```python
from build123d import *

# Parameters (mm, degrees)
BOSS_EXTRUDE1_DEPTH   = 4.7625
F_6_CLEARANCE_HOLE1_D = 4.3053


with BuildPart() as part:
    # Sketch1 → Boss-Extrude1 (new body)
    with BuildSketch(Plane.XY):
        with BuildLine():
            Line((-3103.698757178, 1002.345694712), (-3103.698757178, 1084.895694712))
            Line((-3103.698757178, 1084.895694712), (-3131.638757178, 1084.895694712))
            ThreePointArc((-3131.638757178, 1084.895694712), (-3140.608225903, 1087.139412233), (-3147.464838552, 1093.342032687))
            Line((-3147.464838552, 1093.342032687), (-3159.30564158, 1086.505741871))
            Line((-3159.30564158, 1086.505741871), (-3151.323757178, 1064.575694712))
            Line((-3151.323757178, 1064.575694712), (-3151.323757178, 1045.239932962))
            Line((-3151.323757178, 1045.239932962), (-3126.558757178, 1002.345694712))
            Line((-3126.558757178, 1002.345694712), (-3103.698757178, 1002.345694712))
        make_face()
    extrude(amount=BOSS_EXTRUDE1_DEPTH)

    # #6 Clearance Hole1 (through all)
    with Locations(Plane.XY.offset(4.7625)):
        with Locations((-3122.748757178, 1009.965694712), (-3111.001257178, 1076.958194712)):
            Hole(F_6_CLEARANCE_HOLE1_D / 2)


solid = part.part
```
The listing builds one solid part. Answer for the finished solid, in the listing's coordinates (mm). A direction names the side the tool comes from. Coordinates: 2 decimals unless noted, no trailing zeros. Loops run counter-clockwise (first coordinate to the right, second up) from the corner with the lowest first, then second, coordinate; pieces in that order, holes last. Notation, with made-up numbers: (-18, 59) - (11, 59) arc R6 ccw to (11, 68) - close; hole circle Ø9 at (19.25, -13). An arc over 180 degrees is marked (long way). Write item = value, one per line.
1) Which of the six approach directions +Z, -Z, +X, -X, +Y, -Y give full straight-line access (tool end or side, diameter ignored) to faces 5 (the face through (-3151.324, 1055, 2)), 6 (the face through (-3124.737, 1009.141, 2.348))?
Responses:
face_5 = +Z, -Z, -X, -Y
face_6 = +Z, -Z
2) Find the intervals of material crossed by line 1 along Y through (x, z) = (-3123, 3.1); line 2 along Y through (x, z) = (-3114, 1.75); line 3 along X through (y, z) = (1053.5, 0.45), in increasing order.
Responses:
line_1 = 1002.35 to 1007.83, 1012.1 to 1084.9
line_2 = 1002.35 to 1084.9
line_3 = -3151.32 to -3103.7
3) Section C-C (x = -3107.5) is taken. Determine the outline of the cut face in (y, z).
Responses:
outline = (1002.35, 0) - (1084.9, 0) - (1084.9, 4.76) - (1002.35, 4.76) - close
4) Each of these flat-tipped pins is pushed along its axis until it touches: P1, Ø1, axis at y = 1073.5, z = 3.5, coming from the -X side; P2, Ø10, axis at x = -3141.5, y = 1062, coming from the -Z side; P3, Ø2, axis at x = -3115.5, z = 3.5, coming from the +Y side. Where does it stop, or does it pass through?
Responses:
P1 = -3154.75
P2 = 0
P3 = 1084.9
5) Determine the mould class of faces 1 (the face through (-3140.493, 1087.078, 2.348)), 2 (the face through (-3153.302, 1089.972, 2.348)), 3 (the face through (-3117, 1084.896, 2)), 4 (the face through (-3113.055, 1077.605, 2.348)) for opening direction X: pulls with the +X half, pulls with the -X half, needs draft (parallel to the pull), parting line crosses it, or undercut.
Responses:
face_1 = pulls with the +X half
face_2 = pulls with the -X half
face_3 = needs draft
face_4 = undercut
6) Section A-A (z = 1.8) is taken. Determine the outline of the cut face in (x, y), plus the area to 3 significant figures.
Responses:
outline = (-3159.31, 1086.51) - (-3151.32, 1064.58) - (-3151.32, 1045.24) - (-3126.56, 1002.35) - (-3103.7, 1002.35) - (-3103.7, 1084.9) - (-3131.64, 1084.9) arc R19.05 cw to (-3147.46, 1093.34) - close; hole circle Ø4.31 at (-3122.75, 1009.97); hole circle Ø4.31 at (-3111, 1076.96)
area = 3,550 mm^2
7) Section B-B (y = 1049) is taken. Determine the outline of the cut face in (x, z).
Responses:
outline = (-3151.32, 0) - (-3103.7, 0) - (-3103.7, 4.76) - (-3151.32, 4.76) - close
